For this review, take the finished solid that the model builds, in its own axes (mm). Give positions to 0.01 mm unless a question says otherwise; leave off trailing zeros. Order: outer loops, then holes, each group sorted by start corner. A loop starts at its lowest first (then second) coordinate and runs counter-clockwise, first axis right, second up. Notation, with made-up numbers: (10.5, 17.5) - (35.5, 17.5) arc R28 ccw to (35.5, 40.5) - close; hole circle Ø4 at (20, -17). An arc over 180 degrees is marked (long way). Use a Markdown table: item, result. Add a question column.
1) Clearance check with flat-ended pins moving along their axes: P1, Ø6, axis at x = 18.5, z = -99, coming from the +Y side; P2, Ø1.5, axis at x = 16.5, y = 6.5, coming from the +Z side; P3, Ø2.5, axis at y = 4.08, z = -26.25, coming from the +X side. State where each tip first meets the part, or that it passes through.
2) Wall thickness on L1, parallel to Y at x = 4.5, z = -27; L2, parallel to X at y = 5, z = -22; L3, parallel to Y at x = 16.5, z = -99.75: over which ranges is each line inside the solid? List them lowest first.
3) We need section B-B on x = 5.25. Write out the cut boundary in (y, z).
4) We need section A-A on z = -31. Write out the cut boundary in (x, y).
Autodesk Inventor part; units mm, degrees
ref_plane "Silicone Fitting Plane" through (0, 0, -5.25) normal (0, 0, 1) x (1, 0, 0)
ref_plane "Cap Plane" through (0, 0, -136.5) normal (0, 0, 1) x (1, 0, 0)
ref_plane "YZ Plane" through (0, 0, 0) normal (1, 0, 0) x (0, 1, 0)
ref_plane "Silicone Fitting Plane" through (0, 0, -5.25) normal (0, 0, 1) x (1, 0, 0)
ref_plane "Cap Plane" through (0, 0, -136.5) normal (0, 0, 1) x (1, 0, 0)
sketch "Base Sketch" plane through (0, 0, 0) normal (0, 0, 1) x (1, 0, 0)
  line L0 (0, 0) -> (15, 0)
  line L1 (15, 0) -> (15, 8.1625)
  line L2 (15, 8.1625) -> (0, 8.1625)
  line L3 (0, 8.1625) -> (0, 0)
  line L4 (1.5, 1.5) -> (12, 1.5)
  line L5 (12, 1.5) -> (12, 6.6625)
  line L6 (12, 6.6625) -> (1.5, 6.6625)
  line L7 (1.5, 6.6625) -> (1.5, 1.5)
  dimension "Height" = 8.1625
  dimension "Width" = 15
  dimension "d1" = 1.5
  dimension "d2" = 1.5
  dimension "d3" = 1.5
  dimension "FittingWallWallThickness" = 3
extrude "Base" add sketch "Base Sketch" against normal blind 136.5
sketch "Silicone Fitting Sketch" plane through (0, 0, -5.25) normal (0, 0, 1) x (1, 0, 0)
  line L0 (15, 4.0812) -> (25, 4.0812) construction
  line L1 (25, 4.0812) -> (25, 1.7)
  line L2 (25, 1.7) -> (22, 1)
  line L3 (22, 1) -> (22, 1.7)
  line L4 (22, 1.7) -> (19, 1)
  line L5 (19, 1) -> (19, 1.7)
  line L6 (19, 1.7) -> (15, 1.7)
  line L7 (15, 1.7) -> (15, 4.0812)
  line L8 (25, 1.7) -> (19, 1.7) construction
  line L9 (15, 2.2) -> (25, 2.2)
  line L10 (-5, 0) -> (30, 0) construction
  point P0 (0, 0)
  dimension "FittingLength" = 10
  dimension "FittingRadius" = 2.3813
  dimension "d4" = 0.5
  dimension "BarbHeight" = 0.7
  dimension "BarbLength" = 3
  dimension "d5" = 15
  dimension "FittingClearance" = 1
revolve "Silicone Fitting" add sketch "Silicone Fitting Sketch" angle 360 about axis through (15, 4.0812, -5.25) along (1, 0, 0)
sketch "Airflow Cut Sketch" plane through (15, 4.0812, -5.25) normal (1, 0, 0) x (0, 0, -1)
  circle A0 centre (0, 0) radius 1.8812
  point P0 (-5.25, -4.0812)
extrude "Airflow Cut" cut sketch "Airflow Cut Sketch" against normal up to surface (3 mm away)
pattern_linear "Fitting Repetitions" count 13 spacing 10.5 along (0, 0, -1) of "Silicone Fitting", "Airflow Cut"
sketch "Sketch22" plane through (0, 0, 0) normal (0, 0, 1) x (1, 0, 0)
  line L0 (0.75, 0.75) -> (13.5, 0.75)
  line L1 (13.5, 0.75) -> (13.5, 7.4125)
  line L2 (13.5, 7.4125) -> (0.75, 7.4125)
  line L3 (0.75, 7.4125) -> (0.75, 0.75)
  line L4 (1.5, 1.5) -> (12, 1.5)
  line L5 (12, 1.5) -> (12, 6.6625)
  line L6 (12, 6.6625) -> (1.5, 6.6625)
  line L7 (1.5, 6.6625) -> (1.5, 1.5)
  point P0 (0, 0)
  dimension "d141" = 0.75
  dimension "d142" = 0.75
  dimension "d143" = 6.6625
  dimension "d144" = 12.75
  dimension "d145" = 1.5
  dimension "d146" = 0.75
  dimension "d147" = 0.75
  dimension "d148" = 0.75
extrude "Extrusion21" cut sketch "Sketch22" against normal blind 10.5
sketch "Sketch23" plane through (0, 0, -136.5) normal (0, 0, -1) x (-1, 0, 0)
  line L0 (-12, 1.5) -> (-12, 6.6625)
  line L1 (-12, 6.6625) -> (-1.5, 6.6625)
  line L2 (-1.5, 6.6625) -> (-1.5, 1.5)
  line L3 (-1.5, 1.5) -> (-12, 1.5)
  point P0 (0, 0)
extrude "Extrusion24" add sketch "Sketch23" against normal blind 1.5
equation "\"Height\" = 2 * FittingRadius + 2 * FittingClearance + 2 * BarbHeight"
equation "\"Width\" = ManifoldWidth"
equation "\"d1\" = WallThickness"
equation "\"d2\" = WallThickness"
equation "\"d3\" = WallThickness"
equation "\"FittingWallWallThickness\" = 2 * WallThickness"
equation "\"FittingLength\" = ManifoldFittingLength"
equation "\"d11\" = myKeyWidth + myKeySpacing"
equation "\"d143\" = Height - WallThickness"
equation "\"d144\" = -0.5 * WallThickness + Width - 0.5 * FittingWallWallThickness"
equation "\"d145\" = 0.5 * FittingWallWallThickness"
equation "\"d146\" = 0.5 * WallThickness"
equation "\"d147\" = 0.5 * WallThickness"
equation "\"d148\" = 0.5 * WallThickness"
equation "\"d149\" = KeyWidth + KeySpacing"
equation "\"d155\" = WallThickness"
equation "\"myKeyWidth\" = KeyWidth"
equation "\"myKeySpacing\" = KeySpacing"
equation "\"WallThickness\" = 1.5"
equation "\"d6\" = -0.5 * myKeyWidth - 0.5 * myKeySpacing"
properties part number "ManifoldExtension0" material "ABS Plastic"
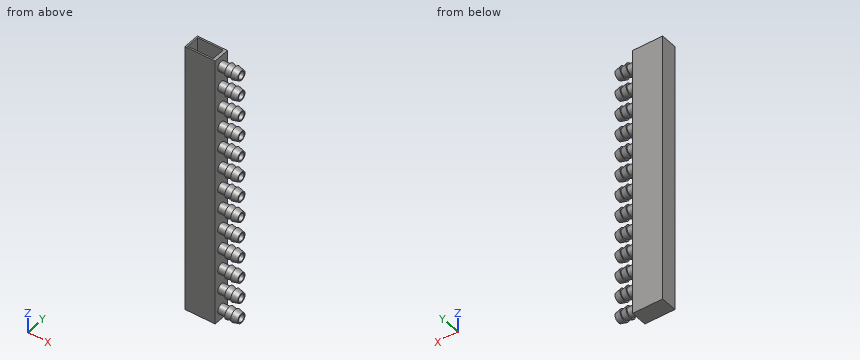
Checked values:
| question | item | result |
|---|---|---|
| 1 | P1 | y = 7.16 |
| 1 | P2 | z = -3.55 |
| 1 | P3 | x = 1.5 |
| 2 | L1 | 0 to 1.5, 6.66 to 8.16 |
| 2 | L2 | 0 to 1.5, 12 to 15 |
| 2 | L3 | 1.7 to 2.2, 5.96 to 6.46 |
| 3 | outline | (0, -136.5) - (8.16, -136.5) - (8.16, 0) - (7.41, 0) - (7.41, -10.5) - (6.66, -10.5) - (6.66, -135) - (1.5, -135) - (1.5, -10.5) - (0.75, -10.5) - (0.75, 0) - (0, 0) - close |
| 4 | outline | (0, 0) - (15, 0) - (15, 8.16) - (0, 8.16) - close; hole (1.5, 1.5) - (12, 1.5) - (12, 6.66) - (1.5, 6.66) - close |
